```python
from build123d import *

# Parameters (mm, degrees)
POCKET_DEPTH = 0.75


with BuildPart() as part:
    # Sketch → Revolution (revolve)
    with BuildSketch(Plane.XZ):
        with BuildLine():
            Line((0, 0), (0, 21.75))
            Line((0, 21.75), (2.25, 21.75))
            ThreePointArc((3, 21), (2.78033, 21.53033), (2.25, 21.75))
            Line((3, 21), (3, 20))
            Line((3, 20), (1.5, 20))
            Line((1.5, 20), (1.5, 0))
            Line((1.5, 0), (0, 0))
        make_face()
    revolve(axis=Axis((0, 0, 0), (0, 0, 1)))

    # Sketch001 (on Face5 of Revolution) → Pocket (cut)
    with BuildSketch(Plane(origin=(0, 0, 21.75), x_dir=(-1, 0, 0), z_dir=(0, 0, 1))):
        Polygon((-3.274783, -2.372712), (2.184691, 3.4031), (3.274783, 2.372712), (-2.184691, -3.4031), align=None)
    extrude(amount=-POCKET_DEPTH, mode=Mode.SUBTRACT)


solid = part.part
```
For this review, take the finished solid that the model builds, in its own axes (mm). A direction names the side the tool comes from. Coordinates: 2 decimals unless noted, no trailing zeros. Loops run counter-clockwise (first coordinate to the right, second up) from the corner with the lowest first, then second, coordinate; pieces in that order, holes last.
1. Add section C-C, the plane z = 7.75. Give the boundary of the cut face in (x, y), then the cut area to 3 significant figures.
2. Insertion check: P1, Ø3, axis at y = 0.5, z = 12, coming from the +X side; P2, Ø1, axis at y = -1.5, z = 11.5, coming from the -X side. Each pin has a flat end and moves straight along its axis. Give the tip position at first contact, or say it passes through.
3. Add section B-B, the plane x = 0. Give the boundary of the cut face in (y, z), then the cut area to 3 significant figures.
4. For line 1 (Z direction, x = 0, y = 1.75); line 2 (Y direction, x = 0, z = 19.25); line 3 (Z direction, x = 2, y = 2), list the stretches that pass through material, from the lowest coordinate up.
5. Add section A-A, the plane y = 0. Give the boundary of the cut face in (x, z), then the cut area to 3 significant figures.
6. For faces 4 (the flat face through (-0.57, 0.49, 21.38)), 5 (the flat face through (-1, 1, 21.75)), 6 (the cylindrical face through (-1.5, 0.07, 9.86)), list the 3-axis set-ups (+Z, -Z, +X, -X, +Y, -Y) from which the entire face can be reached by the end or side of a thin tool; tool diameter is ignored.
7. Mouldability with a two-part tool opening along X and no side actions: class faces 1 (the cylindrical face through (-3, 0.1, 20.5)), 2 (the flat face through (0, 0, 21)), 3 (the flat face through (1.3, -1.3, 20)) as +X half, -X half, draft (parallel to the pull), parting line (faces both ways), or undercut.
Result:
1. outline: circle Ø3 at (0, 0)
1. area: 7.07 mm2
2. P1: stops at x = 1.5
2. P2: stops at x = -1.12
3. outline: (-3, 20) - (-1.5, 20) - (-1.5, 0) - (1.5, 0) - (1.5, 20) - (3, 20) - (3, 21) arc R0.75 ccw to (2.25, 21.75) - (1.09, 21.75) - (1.09, 21) - (-1.09, 21) - (-1.09, 21.75) - (-2.25, 21.75) arc R0.75 ccw to (-3, 21) - close
3. area: 68.6 mm2
4. line 1: z = 20 to 21.75
4. line 2: y = -1.5 to 1.5
4. line 3: z = 20 to 21
5. outline: (-3, 20) - (-1.5, 20) - (-1.5, 0) - (1.5, 0) - (1.5, 20) - (3, 20) - (3, 21) arc R0.75 ccw to (2.25, 21.75) - (1.03, 21.75) - (1.03, 21) - (-1.03, 21) - (-1.03, 21.75) - (-2.25, 21.75) arc R0.75 ccw to (-3, 21) - close
5. area: 68.7 mm2
6. face 4: +Z
6. face 5: +Z, +X, -X, +Y, -Y
6. face 6: -Z
7. face 1: parting line
7. face 2: undercut
7. face 3: draft
